Design review of the part built by this model. Coordinates are the model's own, in mm. A direction names the side the tool comes from. Coordinates: 2 decimals unless noted, no trailing zeros. Order: outer loops, then holes, each group sorted by start corner. A loop starts at its lowest first (then second) coordinate and runs counter-clockwise, first axis right, second up. Notation, with made-up numbers: (-32, 40.25) - (2, 40.25) arc R13 ccw to (2, 63.25) - close; hole circle Ø1 at (6, -23.5). An arc over 180 degrees is marked (long way). Write item = value, one per line. Start each with the question number.
```python
from build123d import *

# Parameters (mm, degrees)
F0_W          = 100
F0_H          = 14
F1_DEPTH      = 25
F2_T          = -3
F3_R          = 4
F3_W          = 5
F3_H          = 5
F4_DEPTH      = 7.001
F4_DEPTH_BACK = 7.001
F5_R          = 3
F6_SIZE       = 0.5
F7_R          = 1


with BuildPart() as f1:
    # F0 (on Top) → F1 (new body)
    with BuildSketch(Plane.XY):
        Rectangle(F0_W, F0_H)
    extrude(amount=F1_DEPTH)

    # F2
    f2_openings = [f1.faces().sort_by_distance(p)[0] for p in [
        (0, 0, 25),
    ]]
    offset(amount=F2_T, openings=f2_openings)

    # F3 (on Front) → F4 (cut, two sides)
    with BuildSketch(Plane.XZ) as f4_sk:
        with Locations((-35, 18)):
            Circle(F3_R)
        with Locations((35, 18)):
            Circle(F3_R)
        with Locations((0, 5.5)):
            Rectangle(F3_W, F3_H)
    extrude(amount=-F4_DEPTH, mode=Mode.SUBTRACT)
    extrude(f4_sk.sketch, amount=F4_DEPTH_BACK, mode=Mode.SUBTRACT)

    # F5
    f5_edges = [f1.edges().sort_by_distance(p)[0] for p in [
        (-50, -7, 12.5),
        (50, -7, 12.5),
        (50, 7, 12.5),
        (-50, 7, 12.5),
    ]]
    fillet(f5_edges, radius=F5_R)

    # F6
    f6_edges = [f1.edges().sort_by_distance(p)[0] for p in [
        (0, 4, 25),
        (0, -4, 25),
        (-47, 0, 25),
        (47, 0, 25),
        (31, 7, 18),
        (39, 5.5, 18),
        (31, 4, 18),
        (31, -4, 18),
        (39, -5.5, 18),
        (31, -7, 18),
        (-39, 7, 18),
        (-31, 5.5, 18),
        (-39, 4, 18),
        (-39, -4, 18),
        (-31, -5.5, 18),
        (-39, -7, 18),
        (-2.5, -4, 5.5),
        (0, -4, 8),
        (2.5, -4, 5.5),
        (-2.5, 4, 5.5),
        (0, 4, 8),
        (2.5, 4, 5.5),
        (-2.5, -7, 5.5),
        (0, -7, 8),
        (2.5, -7, 5.5),
        (0, -7, 3),
        (2.5, 7, 5.5),
        (0, 7, 8),
        (-2.5, 7, 5.5),
        (0, 7, 3),
    ]]
    chamfer(f6_edges, length=F6_SIZE)

    # F7
    f7_edges = [f1.edges().sort_by_distance(p)[0] for p in [
        (-25, 4, 3),
        (-47, 0, 3),
        (-25, -4, 3),
        (25, -4, 3),
        (47, 0, 3),
        (25, 4, 3),
    ]]
    fillet(f7_edges, radius=F7_R)


solid = f1.part
```
Item 1: Add section B-B on y = 0.5. Give the boundary of the cut face in (x, z), plus the area to 3 significant figures.
Item 2: Add section C-C on x = -18.5. Give the boundary of the cut face in (y, z).
Item 3: For faces 1 (the cylindrical face through (-37.95, -5.49, 20.7)), 2 (the flat face through (-1, 4, 14)), list the 3-axis set-ups (+Z, -Z, +X, -X, +Y, -Y) from which the entire face can be reached by the end or side of a thin tool; tool diameter is ignored.
Item 4: Add section D-D on z = 18. State how many separate pieces and enclosed holes the cut face has, plus the area to 3 significant figures.
Item 5: For line 1 (X direction, y = -0.75, z = 8.75); line 2 (Z direction, x = -35, y = 5.25); line 3 (Y direction, x = -3.5, z = 11.25), list the stretches that pass through material, from the lowest coordinate up.
Item 6: Mouldability with a two-part tool opening along Z and no side actions: class faces 3 (the flat face through (47, 0, 14)), 4 (the flat face through (-1, 5, 25)), 5 (the flat face through (-2.5, -5, 5)), 6 (the flat face through (0, 5, 8)) as +Z half, -Z half, draft (parallel to the pull), parting line (faces both ways), or undercut.
Item 7: Add section A-A on x = 1.5. Give the boundary of the cut face in (y, z).
Item 8: For P1, Ø1, axis at y = 5, z = 4.5, coming from the +X side; P2, Ø2, axis at y = -6, z = 6, coming from the -X side; P3, Ø1, axis at y = -6, z = 4.5, coming from the +X side, all flat-tipped, find the tip position at first contact; note any pin that passes through.
Worked out:
q1.outline = (-50, 0) - (50, 0) - (50, 25) - (47.5, 25) - (47, 24.5) - (47, 4) arc R1 cw to (46, 3) - (-46, 3) arc R1 cw to (-47, 4) - (-47, 24.5) - (-47.5, 25) - (-50, 25) - close
q1.area = 432 mm2
q2.outline = (-7, 0) - (7, 0) - (7, 25) - (4.5, 25) - (4, 24.5) - (4, 4) arc R1 cw to (3, 3) - (-3, 3) arc R1 cw to (-4, 4) - (-4, 24.5) - (-4.5, 25) - (-7, 25) - close
q3.face_1 = +Y, -Y
q3.face_2 = +Z
q4.separate_pieces = 4
q4.enclosed_holes = 0
q4.area = 542 mm2
q5.line_1 = -50 to -47, 47 to 50
q5.line_2 = 0 to 14, 22 to 25
q5.line_3 = -7 to -4, 4 to 7
q6.face_3 = draft
q6.face_4 = +Z half
q6.face_5 = undercut
q6.face_6 = undercut
q7.outline = (-7, 0) - (7, 0) - (7, 2.5) - (6.5, 3) - (-6.5, 3) - (-7, 2.5) - close; (-7, 8.5) - (-6.5, 8) - (-4.5, 8) - (-4, 8.5) - (-4, 24.5) - (-4.5, 25) - (-7, 25) - close; (4, 8.5) - (4.5, 8) - (6.5, 8) - (7, 8.5) - (7, 25) - (4.5, 25) - (4, 24.5) - close
q8.P1 = 49.96
q8.P2 = -49.83
q8.P3 = 49.6
